Model file for the job. Use its own axes, mm. Round coordinates to 2 decimals unless told otherwise and drop trailing zeros. Loops run counter-clockwise (first coordinate to the right, second up) from the corner with the lowest first, then second, coordinate; pieces in that order, holes last. Notation, with made-up numbers: M 21.25,76 L 26.25,76 A5 ccw 26.25,82 Z; hole C 74,89.25 d9. An arc over 180 degrees is marked long. Use a Markdown table: item, result. Add a question column.
Q1. Pin check, flat tips, straight feed: pin 1 (1.5 mm diameter, centred on x = -0.5, z = 5.5, fed in from +Y); pin 2 (6 mm diameter, centred on x = -0.5, z = 7.5, fed in from +Y). Stop position of each tip, or through.
Q2. Probe line 1 (Y direction, x = 5.75, z = 7.5); line 2 (X direction, y = 14.25, z = 5.5); line 3 (Z direction, x = 1.5, y = 17.5). List the from-to ranges inside material, lowest first. Write a range as from..to.
Q3. Cut at C-C (z = -0.75). Give the cut face in (x, y), plus the area to 3 significant figures.
Q4. Cut at B-B (y = 17). Give the cut face in (x, z), plus the area to 3 significant figures.
Q5. Cut at A-A (z = 3.5). Give the cut face in (x, y).
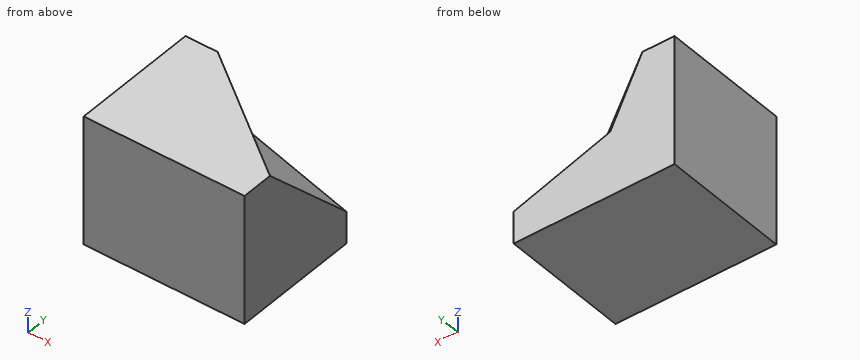
from build123d import *

# Parameters (mm, degrees)
SKETCH_1_W          = 25
SKETCH_1_H          = 20
EXTRUDE_1_DEPTH     = 20
CUT_EXTRUDE_1_DEPTH = 20
CUT_EXTRUDE_5_DEPTH = 20


with BuildPart() as part:
    # 草圖1 → 填料-伸長1 (new body)
    with BuildSketch(Plane(origin=(0, 0, 0), x_dir=(1, 0, 0), z_dir=(0, 1, 0))):
        Rectangle(SKETCH_1_W, SKETCH_1_H)
    extrude(amount=EXTRUDE_1_DEPTH)

    # 草圖5 → 除料-伸長1 (cut)
    with BuildSketch(Plane(origin=(7.981651376, 10.642201835, 3.990825688), x_dir=(-0.818367137, 0.538104419, 0.201789157), z_dir=(-0.574695771, -0.766261028, -0.287347886))):
        Polygon((-5.521175546, -7.607674568), (18.917733471, -2.340822944), (12.808006217, 7.022468832), align=None)
    extrude(amount=-CUT_EXTRUDE_1_DEPTH, mode=Mode.SUBTRACT)

    # 草圖7 → 除料-伸長5 (cut)
    with BuildSketch(Plane(origin=(3.026315789, 9.078947368, 9.078947368), x_dir=(0.973328527, -0.162221421, -0.162221421), z_dir=(0.229415734, 0.688247202, 0.688247202))):
        Polygon((9.733285268, -3.535533906), (9.733285268, 17.67766953), (-5.67774974, 14.142135624), align=None)
    extrude(amount=CUT_EXTRUDE_5_DEPTH, mode=Mode.SUBTRACT)


solid = part.part
Checked values:
| question | item | result |
|---|---|---|
| 1 | pin 1 | stops at y = 17.07 |
| 1 | pin 2 | stops at y = 18.2 |
| 2 | line 1 | y = 0..11 |
| 2 | line 2 | x = -12.5..2.42 |
| 2 | line 3 | z = -10..1.17 |
| 3 | outline | M -12.5,0 L 12.5,0 L 12.5,15.75 L -0.25,20 L -12.5,20 Z |
| 3 | area | 473 mm^2 |
| 4 | outline | M -12.5,-10 L 12.5,-10 L 12.5,-2 L 0.5,2 L -3.5,10 L -12.5,10 Z |
| 4 | area | 364 mm^2 |
| 5 | outline | M -12.5,0 L 12.5,0 L 12.5,11.5 L 2.75,14.75 L -4.25,20 L -12.5,20 Z |
